Design review of the part built by this model. Coordinates are the model's own, in mm. Coordinates: 2 decimals unless noted, no trailing zeros. Write each loop counter-clockwise with the first axis right and the second up, starting at its lowest first coordinate (ties: lowest second). Pieces come first, ordered by that corner, then holes. Notation, with made-up numbers: (56, 12.25) -> (109, 12.25) arc R23 ccw to (109, 35.25) -> close; hole circle Ø9 at (74.5, 64.25). An arc over 180 degrees is marked (long way). Write item = value, one per line. Start each with the question number.
Autodesk Inventor part; units mm, degrees
ref_plane "YZ Plane" through (0, 0, 0) normal (1, 0, 0) x (0, 1, 0)
ref_plane "XZ Plane" through (0, 0, 0) normal (0, 1, 0) x (-1, 0, 0)
ref_plane "XY Plane" through (0, 0, 0) normal (0, 0, 1) x (1, 0, 0)
sketch "Sketch1" plane through (0, 0, 0) normal (0, 0, 1) x (1, 0, 0)
  line L0 (5, -3) -> (23, -3)
  line L1 (28, 2) -> (28, 2)
  line L2 (23, 7) -> (5, 7)
  line L3 (0, 2) -> (0, 2)
  arc A0 (5, 7) -> (0, 2) centre (5, 2) ccw
  arc A1 (0, 2) -> (5, -3) centre (5, 2) ccw
  arc A2 (28, 2) -> (23, 7) centre (23, 2) ccw
  arc A3 (23, -3) -> (28, 2) centre (23, 2) ccw
  circle A4 centre (5, 2) radius 1.5
  circle A5 centre (23, 2) radius 1.5
  point P0 (0, -3)
  point P1 (28, -3)
  point P2 (0, 7)
  dimension "d0" = 28
  dimension "d1" = 10
  dimension "d2" = 5
  dimension "d4" = 3
  dimension "d5" = 3
extrude "Extrusion1" add sketch "Sketch1" along normal blind 3
properties part number "plastic_part_5"
(1) For pin 1 Ø3.5 at (x, y) = (5, 2) entering from -Z; pin 2 Ø2.5 at (x, y) = (23, 2) entering from +Z; pin 3 Ø1.5 at (y, z) = (3, 2) entering from +X, all flat-tipped, find the tip position at first contact; note any pin that passes through.
(2) Take a section at A-A, the plane y = 2. State the section outline as (x, z) points.
(3) Take a section at D-D, the plane y = -1. State the section outline as (x, z) points.
(4) Take a section at C-C, the plane z = 1.95. State the section outline as (x, y) points.
(5) For line 1 (Y direction, x = 23, z = 2.8); line 2 (X direction, y = 1, z = 1.1); line 3 (X direction, y = -0.25, z = 1.1), list the stretches that pass through material, from the lowest coordinate up.
(6) Mouldability with a two-part tool opening along X and no side actions: class faces 1 (the face through (14, 2, 3)), 2 (the face through (0, 2, 1)), 3 (the face through (5.806, 0.735, 1.479)) as pulls with the +X half, pulls with the -X half, needs draft (parallel to the pull), parting line crosses it, or undercut.
(7) Take a section at B-B, the plane x = 4. State the section outline as (y, z) points, then the cut area to 3 significant figures.
Report:
q1.pin_1 = 0
q1.pin_2 = through
q1.pin_3 = 27.99
q2.outline = (0, 0) -> (3.5, 0) -> (3.5, 3) -> (0, 3) -> close; (6.5, 0) -> (21.5, 0) -> (21.5, 3) -> (6.5, 3) -> close; (24.5, 0) -> (28, 0) -> (28, 3) -> (24.5, 3) -> close
q3.outline = (1, 0) -> (27, 0) -> (27, 3) -> (1, 3) -> close
q4.outline = (5, -3) -> (23, -3) arc R5 ccw to (23, 7) -> (5, 7) arc R5 ccw to start; hole circle Ø3 at (5, 2); hole circle Ø3 at (23, 2)
q5.line_1 = -3 to 0.5, 3.5 to 7
q5.line_2 = 0.1 to 3.88, 6.12 to 21.88, 24.12 to 27.9
q5.line_3 = 0.53 to 27.47
q6.face_1 = needs draft
q6.face_2 = pulls with the -X half
q6.face_3 = undercut
q7.outline = (-2.9, 0) -> (0.88, 0) -> (0.88, 3) -> (-2.9, 3) -> close; (3.12, 0) -> (6.9, 0) -> (6.9, 3) -> (3.12, 3) -> close
q7.area = 22.7 mm2
